Autodesk Inventor part; units mm, degrees
sketch "Boceto1" plane through (0, 0, 0) normal (0, 0, 1) x (1, 0, 0)
  line L0 (10, -10) -> (-10, -10)
  line L1 (-10, -10) -> (-10, 10)
  line L2 (-10, 10) -> (10, 10)
  line L3 (10, 10) -> (10, -10)
  line L4 (10, -10) -> (-10, 10) construction
  line L5 (-10, -10) -> (10, 10) construction
  line L6 (2.55, 6) -> (-2.55, 6) construction
  line L7 (-2.55, 6) -> (2.55, 6)
  line L8 (2.55, 6) -> (2.55, -2.6)
  line L9 (2.55, -2.6) -> (-2.55, -2.6)
  line L10 (-2.55, -2.6) -> (-2.55, 6)
  point P0 (0, 0)
  point P1 (0, 6)
  dimension "d0" = 20
  dimension "d1" = 4
  dimension "d2" = 5.1
  dimension "d3" = 8.6
extrude "Extrusión1" add sketch "Boceto1" along normal mid plane 3
sketch "Boceto2" plane through (0, 0, 1.5) normal (0, 0, 1) x (1, 0, 0)
  line L0 (10, 10) -> (-10, 10)
  line L1 (-10, -10) -> (10, -10)
  line L2 (-7.5, 10) -> (-5, 10)
  line L3 (-5, 10) -> (-5, -10)
  line L4 (-5, -10) -> (-7.5, -10)
  line L5 (-7.5, -10) -> (-7.5, 10)
  line L6 (5, 10) -> (7.5, 10)
  line L7 (7.5, 10) -> (7.5, -10)
  line L8 (7.5, -10) -> (5, -10)
  line L9 (5, -10) -> (5, 10)
  line L10 (0, -14) -> (0, 14)
  point P0 (0, 0)
  point P1 (-5, 10)
  point P2 (5, -10)
  dimension "d6" = 2.5
  dimension "d7" = 5
extrude "Extrusión2" cut sketch "Boceto2" against normal blind 1.5 contours L7 L1 L9 L0 | L3 L1 L5 L0
sketch "Boceto5" plane through (-10, -10, -1.5) normal (0, -1, 0) x (1, 0, 0)
  line L0 (20, -17) -> (0, -17)
  line L1 (0, -17) -> (0, 3)
  line L2 (0, 3) -> (20, 3)
  line L3 (20, 3) -> (20, -17)
  line L4 (20, -17) -> (0, 3) construction
  line L5 (0, -17) -> (20, 3) construction
  line L6 (12.5, -4.5) -> (7.5, -4.5) construction
  line L7 (7.5, -4.5) -> (12.5, -4.5)
  line L8 (12.5, -4.5) -> (12.5, -13)
  line L9 (12.5, -13) -> (7.5, -13)
  line L10 (7.5, -13) -> (7.5, -4.5)
  point P0 (10, 1.5)
  point P1 (10, -7)
  point P2 (10, -4.5)
  dimension "d12" = 20
  dimension "d14" = 5
  dimension "d15" = 8.5
  dimension "d16" = 4
extrude "Extrusión3" add sketch "Boceto5" against normal blind 3
sketch "Boceto6" plane through (-10, -10, 1.5) normal (0, -1, 0) x (1, 0, 0)
  line L0 (0, -20) -> (20, -20)
  line L1 (15, 0) -> (5, 0)
  line L2 (17.5, -20) -> (15, -20)
  line L3 (15, -20) -> (15, 0)
  line L4 (15, 0) -> (17.5, 0)
  line L5 (17.5, 0) -> (17.5, -20)
  line L6 (7.5, -7.5) -> (12.5, -7.5)
  line L7 (2.5, 0) -> (5, 0)
  line L8 (5, -20) -> (2.5, -20)
  line L9 (2.5, -20) -> (2.5, 0)
  line L10 (2.5, 0) -> (5, 0)
  line L11 (5, 0) -> (5, -20)
  line L12 (10, -24) -> (10, 4)
  point P0 (10, -1.5)
  point P1 (10, -7.5)
  point P2 (10, -7.5)
  point P3 (2.5, -20)
  dimension "d19" = 2.5
  dimension "d20" = 5
extrude "Extrusión4" cut sketch "Boceto6" against normal blind 1.5 contours L9 L7 L11 L0 | L3 L4 L5 L0
sketch "Boceto7" plane through (10, -10, 1.5) normal (1, 0, 0) x (0, 0, -1)
  line L0 (0, 20) -> (3, 20)
  line L1 (20, 0) -> (20, 3)
  line L2 (3, 20) -> (20, 3)
  line L3 (20, 3) -> (3, 3)
  line L4 (3, 3) -> (3, 20)
  point P0 (1.5, 10)
extrude "Extrusión5" add sketch "Boceto7" against normal blind 1.5
mirror "Simetría1" about plane through (0, 0, 0) normal (1, 0, 0) of "Extrusión5"
properties part number "Soporte_2020_0001"
Check sheet for the modelled part. Datum: model origin and axes. Units: mm. A direction names the side the tool comes from. Round coordinates to 2 decimals unless told otherwise and drop trailing zeros. Order: outer loops, then holes, each group sorted by start corner. A loop starts at its lowest first (then second) coordinate and runs counter-clockwise, first axis right, second up.
1) Section check B-B (y = 5). Record the boundary of the cut face in (x, z).
2) Scan lines: line 1 (X direction, y = 2.75, z = -8); line 2 (X direction, y = -7.25, z = -6.25); line 3 (Y direction, x = 0, z = -0.5). Record each from-to range of solid material in increasing order.
3) Tool access check on faces 4 (the flat face through (5, 1, 1)), 5 (the flat face through (5, -9, -9)), 6 (the flat face through (-8.5, -2, -6)). Record the directions out of +Z, -Z, +X, -X, +Y, -Y that give a thin tool (end or side, any length) a straight path to the whole face; none if there is none.
4) Section check C-C (x = -1). Record the boundary of the cut face in (y, z), and give its area (3 significant figures).
5) Go/stop test with a flat-tipped pin: pin 1 Ø4 at (y, z) = (2.5, -13) entering from +X. Record where the tip stops, or that it passes through.
6) Section check D-D (y = -8). Record the boundary of the cut face in (x, z).
7) Mould release check, pull along Y, two halves, no side actions. Record for faces 1 (the flat face through (-7.5, 1, 1)), 2 (the flat face through (0, -2.6, 0)), 3 (the flat face through (-6, -8.5, -8)): +Y half, -Y half, draft (parallel to the pull), parting line (faces both ways), or undercut.
8) Section check A-A (z = -12.5). Record the boundary of the cut face in (x, y), and give its area (3 significant figures).
Result:
1. outline: (-10, -6.5) - (-8.5, -6.5) - (-8.5, -1.5) - (-2.55, -1.5) - (-2.55, 1.5) - (-5, 1.5) - (-5, 0) - (-7.5, 0) - (-7.5, 1.5) - (-10, 1.5) - close; (2.55, -1.5) - (8.5, -1.5) - (8.5, -6.5) - (10, -6.5) - (10, 1.5) - (7.5, 1.5) - (7.5, 0) - (5, 0) - (5, 1.5) - (2.55, 1.5) - close
2. line 1: x = -10 to -8.5, 8.5 to 10
2. line 2: x = -10 to -2.5, 2.5 to 10
2. line 3: y = -10 to -2.6, 6 to 10
3. face 4: +Z, +Y
3. face 5: +Z, -Z, -Y
3. face 6: -Z, +Y
4. outline: (-10, -18.5) - (-7, -18.5) - (-7, -14.5) - (-10, -14.5) - close; (-10, -6) - (-7, -6) - (-7, -1.5) - (-2.6, -1.5) - (-2.6, 1.5) - (-10, 1.5) - close; (6, -1.5) - (10, -1.5) - (10, 1.5) - (6, 1.5) - close
4. area: 59.7 mm2
5. pin 1: passes through
6. outline: (-10, -18.5) - (10, -18.5) - (10, 1.5) - (-10, 1.5) - close; hole (-2.5, -14.5) - (2.5, -14.5) - (2.5, -6) - (-2.5, -6) - close
7. face 1: draft
7. face 2: undercut
7. face 3: -Y half
8. outline: (-10, -10) - (-7.5, -10) - (-7.5, -8.5) - (-5, -8.5) - (-5, -10) - (-2.5, -10) - (-2.5, -7) - (-8.5, -7) - (-8.5, -1) - (-10, -1) - close; (2.5, -10) - (5, -10) - (5, -8.5) - (7.5, -8.5) - (7.5, -10) - (10, -10) - (10, -1) - (8.5, -1) - (8.5, -7) - (2.5, -7) - close
8. area: 55.5 mm2
